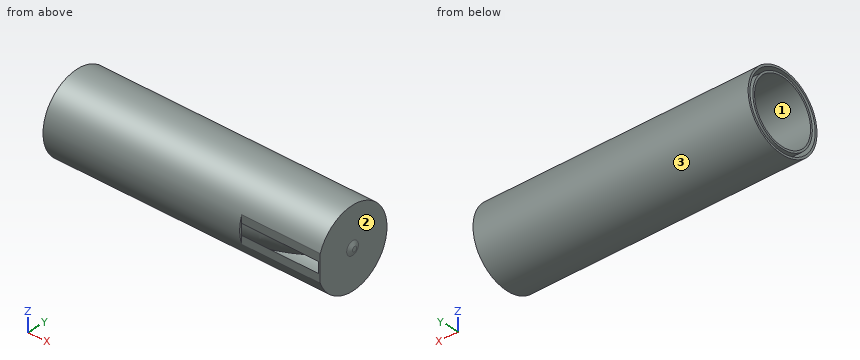
```python
from build123d import *

# Parameters (mm, degrees)
IZIM3_R                     = 33.579638097
Y_KSEKLIK_EKSTR_ZYON1_DEPTH = 10
Y_KSEKLIK_EKSTR_ZYON1_TAPER = 65
KES_EKSTR_ZYON1_START       = 1000
KES_EKSTR_ZYON1_DEPTH       = 436
KES_EKSTR_ZYON2_DEPTH       = 729


with BuildPart() as part:
    # Çizim1 → Döndür2 (revolve)
    with BuildSketch(Plane.XY, mode=Mode.PRIVATE) as d_nd_r2_sk:
        with BuildLine():
            Line((0, 160), (800, 160))
            ThreePointArc((800, 160), (1108.966687108, 121.793262795), (1399.319473661, 9.474841102))
            Line((1399.319473661, 9.474841102), (1399.319473661, 196.645479286))
            Line((1399.319473661, 196.645479286), (0, 196.645479286))
            Line((0, 196.645479286), (0, 160))
        make_face()
    revolve(d_nd_r2_sk.sketch.rotate(Axis((0, 0, 0), (1, 0, 0)), 180), axis=Axis((0, 0, 0), (1, 0, 0)))

    # Çizim2 → Kes-Döndür1 (revolve, cut)
    with BuildSketch(Plane.XY, mode=Mode.PRIVATE) as kes_d_nd_r1_sk:
        with BuildLine():
            Line((1389.319473661, 26.059788693), (1389.319473661, 186.645479286))
            Line((1389.319473661, 186.645479286), (-316.134237936, 186.645479286))
            Line((-316.134237936, 186.645479286), (-316.134237936, 170))
            Line((-316.134237936, 170), (800, 170))
            ThreePointArc((800, 170), (1103.321704823, 133.493691238), (1389.319473661, 26.059788693))
        make_face()
    revolve(kes_d_nd_r1_sk.sketch.rotate(Axis((0, 0, 0), (1, 0, 0)), 180), axis=Axis((0, 0, 0), (1, 0, 0)), mode=Mode.SUBTRACT)

    # Çizim3 → Yükseklik-Ekstrüzyon1 (add)
    with BuildSketch(Plane(origin=(1399.319473661, 0, 0), x_dir=(0, 0, -1), z_dir=(1, 0, 0))):
        Circle(IZIM3_R)
    extrude(amount=Y_KSEKLIK_EKSTR_ZYON1_DEPTH, taper=Y_KSEKLIK_EKSTR_ZYON1_TAPER)

    # Çizim4 → Kes-Ekstrüzyon1 (cut)
    with BuildSketch(Plane(origin=(0, 0, 0), x_dir=(0, 0, -1), z_dir=(1, 0, 0)).offset(KES_EKSTR_ZYON1_START)):
        Polygon((97.176759239, -191.217657376), (-137.732913501, -191.217657376), (-99.977691978, -250.955991759), (64.615874303, -223.778542312), align=None)
    extrude(amount=KES_EKSTR_ZYON1_DEPTH, mode=Mode.SUBTRACT)

    # Çizim5 → Kes-Ekstrüzyon2 (cut)
    with BuildSketch(Plane(origin=(1000, 0, 0), x_dir=(0, 0, -1), z_dir=(1, 0, 0))):
        Polygon((-78.243246347, -184.594850552), (94.834250253, -184.594850552), (68.709345106, -210.7197557), (-83.685934919, -208.179834366), align=None)
    extrude(amount=KES_EKSTR_ZYON2_DEPTH, mode=Mode.SUBTRACT)


solid = part.part
```
CAD build for the part. Positions are in the model's coordinates, mm. Face numbers are marked on the shaded views. Give positions to 0.01 mm unless a question says otherwise; leave off trailing zeros. Loops run counter-clockwise (first coordinate to the right, second up) from the corner with the lowest first, then second, coordinate; pieces in that order, holes last. Notation, with made-up numbers: (-27.75, -1) - (-13.75, -1) arc R28 ccw to (-13.75, 24) - close; hole circle Ø5 at (28, -30.5). An arc over 180 degrees is marked (long way). Put each result on its own line as item: value.
Q1. Slice it at A-A (x = 670). Give the cut face in (y, z), plus the area to 3 significant figures.
Filled in:
outline: circle Ø393.29 at (0, 0); circle Ø340 at (0, 0); hole circle Ø373.29 at (0, 0); hole circle Ø320 at (0, 0)
area: 22,400 mm²
Q2. Flat gauge pins, fed straight in: pin 1 (8 mm diameter, centred on x = 408.5, z = 127.5, fed in from -Y); pin 2 (10 mm diameter, centred on y = -72.5, z = -140.5, fed in from +X); pin 3 (3 mm diameter, centred on x = 185, y = 86, fed in from +Z). Where does each tip first touch, or does it go through?
Filled in:
pin 1: stops at y = -153.03
pin 2: stops at x = 1399.32
pin 3: stops at z = 177.56
Q3. Probe line 1 along Z through (x, y) = (494.5, 0); line 2 along Z through (x, y) = (126, -9.5); line 3 along Y through (x, z) = (378.5, 42). List the from-to ranges inside material, lowest first.
Filled in:
line 1: z = -196.65 to -186.65, -170 to -160, 160 to 170, 186.65 to 196.65
line 2: z = -196.42 to -186.4, -169.73 to -159.72, 159.72 to 169.73, 186.4 to 196.42
line 3: y = -192.11 to -181.86, -164.73 to -154.39, 154.39 to 164.73, 181.86 to 192.11
Q4. Slice it at B-B (x = 1311.5). Give the number of separate pieces and of enclosed holes in the cut face, plus the area to 3 significant figures.
Filled in:
separate pieces: 2
enclosed holes: 1
area: 15,000 mm²
Q5. Mould opens along Y. For the marked faces 1, 2 and 3 say: pulls with the +Y half, pulls with the -Y half, needs draft (parallel to the pull), parting line crosses it, or undercut.
Filled in:
face 1: undercut
face 2: needs draft
face 3: parting line crosses it
